Work out the finished part from the listing and answer in its coordinate system (mm). Give positions to 0.01 mm unless a question says otherwise; leave off trailing zeros. Write each loop counter-clockwise with the first axis right and the second up, starting at its lowest first coordinate (ties: lowest second). Pieces come first, ordered by that corner, then holes. Notation, with made-up numbers: (82, 12) -> (137, 12) arc R34 cw to (137, 45) -> close; hole circle Ø11 at (83, 30). An arc over 180 degrees is marked (long way). Use a Markdown table: item, result. Add a question column.
Q1. Consider line 1 (Y direction, x = 1.3, z = -26.5); line 2 (Z direction, x = 2.3, y = 66.5). Determine where each line is inside the solid, lowest interval first.
Q2. Section B-B, the plane y = -65.5 is taken. Give the vertices of the cut face in (x, z), plus the area to 3 significant figures.
Q3. Each of these flat-tipped pins is pushed along its axis until it touches: pin 1 Ø0.9 at (x, y) = (1.5, 7) entering from +Z; pin 2 Ø1.5 at (x, y) = (1.5, 147.5) entering from -Z. Where does it stop, or does it pass through?
Q4. Section A-A, the plane x = 2.35 is taken. State how many separate pieces and enclosed holes the cut face has, plus the area to 4 significant figures.
from build123d import *

# Parameters (mm, degrees)
SKETCH_1_W      = 20
SKETCH_1_H      = 3
EXTRUDE_5_DEPTH = 3


with BuildPart() as part:
    # Эскиз1 → Бобышка-Вытянуть5 (new body)
    with BuildSketch(Plane(origin=(0, 0, 0), x_dir=(0, 0, -1), z_dir=(1, 0, 0))):
        Polygon((-69.5, -165), (-69.5, -145), (-66.5, -145), (-66.5, -125), (-69.5, -125), (-69.5, -75), (-66.5, -75), (-66.5, -55), (-69.5, -55), (-69.5, -5), (-66.5, -5), (-66.5, 15), (-69.5, 15), (-69.5, 65), (-66.5, 65), (-66.5, 85), (-69.5, 85), (-69.5, 135), (-66.5, 135), (-66.5, 155), (-69.5, 155), (-69.5, 165), (69.5, 165), (69.5, 155), (66.5, 155), (66.5, 135), (69.5, 135), (69.5, 85), (66.5, 85), (66.5, 65), (69.5, 65), (69.5, 15), (66.5, 15), (66.5, -5), (69.5, -5), (69.5, -55), (66.5, -55), (66.5, -75), (69.5, -75), (69.5, -125), (66.5, -125), (66.5, -145), (69.5, -145), (69.5, -165), align=None)
        with Locations((25.5, -85.5)):
            Rectangle(SKETCH_1_W, SKETCH_1_H, mode=Mode.SUBTRACT)
        with Locations((-25.5, -85.5)):
            Rectangle(SKETCH_1_W, SKETCH_1_H, mode=Mode.SUBTRACT)
    extrude(amount=EXTRUDE_5_DEPTH)


solid = part.part
Result set:
| question | item | result |
|---|---|---|
| 1 | line 1 | y = -165 to -87, -84 to 165 |
| 1 | line 2 | z = -66.5 to 66.5 |
| 2 | outline | (0, -66.5) -> (3, -66.5) -> (3, 66.5) -> (0, 66.5) -> close |
| 2 | area | 399 mm2 |
| 3 | pin 1 | stops at z = 66.5 |
| 3 | pin 2 | stops at z = -66.5 |
| 4 | separate pieces | 1 |
| 4 | enclosed holes | 2 |
| 4 | area | 45,150 mm2 |
